from build123d import *

# Parameters (mm, degrees)
THREAD_START          = -5
SKETCH1_R             = 6
THREAD_DEPTH          = 5
LOCK_NUT_START        = -8
SKETCH2_R             = 8.5
LOCK_NUT_DEPTH        = 3
SKETCH3_R             = 8.5
BODY_DEPTH            = 6
DOME_START            = 6
SKETCH4_R             = 6.5
DOME_DEPTH            = 8
CABLE_HOLE_DEPTH      = 19.452642087
CABLE_HOLE_DEPTH_BACK = 19.452642087
SKETCH5_R             = 2.5


with BuildPart() as part:
    # Sketch1 → Thread (new body)
    with BuildSketch(Plane.XY.offset(THREAD_START)):
        Circle(SKETCH1_R)
    extrude(amount=THREAD_DEPTH)

    # Sketch2 → Lock_Nut (add)
    with BuildSketch(Plane.XY.offset(LOCK_NUT_START)):
        Circle(SKETCH2_R)
    extrude(amount=LOCK_NUT_DEPTH)

    # Sketch3 → Body (add)
    with BuildSketch(Plane.XY):
        Circle(SKETCH3_R)
    extrude(amount=BODY_DEPTH)

    # Sketch4 → Dome (add)
    with BuildSketch(Plane.XY.offset(DOME_START)):
        Circle(SKETCH4_R)
    extrude(amount=DOME_DEPTH)

    # Sketch5 → Cable_Hole (cut, two sides: drawn at the far end of the back side and taken through both)
    with BuildSketch(Plane.XY.offset(-CABLE_HOLE_DEPTH_BACK)):
        Circle(SKETCH5_R)
    extrude(amount=CABLE_HOLE_DEPTH + CABLE_HOLE_DEPTH_BACK, mode=Mode.SUBTRACT)


solid = part.part
Geometry check sheet. Reference: the model listing, model coordinates, mm. A direction names the side the tool comes from. Give positions to 0.01 mm unless a question says otherwise; leave off trailing zeros. Order: outer loops, then holes, each group sorted by start corner. A loop starts at its lowest first (then second) coordinate and runs counter-clockwise, first axis right, second up. Notation, with made-up numbers: (61.5, 40.25) - (110.5, 40.25) arc R35 ccw to (110.5, 74.25) - close; hole circle Ø2 at (6, 15). An arc over 180 degrees is marked (long way). Use one line per item in the form item = value.
1) Sectioned sample at C-C (z = 11.75). Record the boundary of the cut face in (x, y).
Working result:
outline = circle Ø13 at (0, 0); hole circle Ø5 at (0, 0)
2) Material ranges on probe 1 along Z at (x, y) = (5.25, 3.5); probe 2 along Y at (x, z) = (0, 8); probe 3 along Z at (x, y) = (1.75, -7), recorded low to high. Write a range as from..to.
Working result:
probe_1 = -8..-5, 0..14
probe_2 = -6.5..-2.5, 2.5..6.5
probe_3 = -8..-5, 0..6
3) Sectioned sample at D-D (x = 4.5). Record the boundary of the cut face in (y, z), and give its area (3 significant figures).
Working result:
outline = (-7.21, -8) - (7.21, -8) - (7.21, -5) - (3.97, -5) - (3.97, 0) - (7.21, 0) - (7.21, 6) - (4.69, 6) - (4.69, 14) - (-4.69, 14) - (-4.69, 6) - (-7.21, 6) - (-7.21, 0) - (-3.97, 0) - (-3.97, -5) - (-7.21, -5) - close
area = 245 mm^2
4) Draft check along Z on faces 4 (the face through (2, 6, 0)), 5 (the face through (4.57, 7.167, -6.521)), 6 (the face through (2, -2, -8)). Enter one of: released by +Z, released by -Z, zero draft, split by the parting line, or undercut.
Working result:
face_4 = undercut
face_5 = zero draft
face_6 = released by -Z
5) Depth check by flat-ended pin: pin 1 Ø5 at (x, z) = (-3.5, 3.5) entering from +Y; pin 2 Ø3 at (y, z) = (3, 5.5) entering from -X; pin 3 Ø3 at (x, y) = (0, 0) entering from +Z; pin 4 Ø1.5 at (y, z) = (-6, 11.5) entering from +X. Enter the tip coordinate at first touch or a pass-through.
Working result:
pin_1 = 8.44
pin_2 = -8.37
pin_3 = through
pin_4 = 3.83
6) Sectioned sample at A-A (y = 0). Record the boundary of the cut face in (x, z), and give its area (3 significant figures).
Working result:
outline = (-8.5, -8) - (-2.5, -8) - (-2.5, 14) - (-6.5, 14) - (-6.5, 6) - (-8.5, 6) - (-8.5, 0) - (-6, 0) - (-6, -5) - (-8.5, -5) - close; (2.5, -8) - (8.5, -8) - (8.5, -5) - (6, -5) - (6, 0) - (8.5, 0) - (8.5, 6) - (6.5, 6) - (6.5, 14) - (2.5, 14) - close
area = 207 mm^2
7) Access from +Z, -Z, +X, -X, +Y, -Y to the whole of each face (thin tool, end or side, straight path). Record for faces 1 (the face through (-0.54, -2.44, 2.85)), 2 (the face through (4.4, -5, 6)), 3 (the face through (-6, 0, -3)).
Working result:
face_1 = +Z, -Z
face_2 = +Z
face_3 = none
